Check sheet for the modelled part. Datum: model origin and axes. Units: mm. A direction names the side the tool comes from. Coordinates: 2 decimals unless noted, no trailing zeros. Loops run counter-clockwise (first coordinate to the right, second up) from the corner with the lowest first, then second, coordinate; pieces in that order, holes last. Notation, with made-up numbers: (25.25, 9.25) -> (74.25, 9.25) arc R10 cw to (74.25, 13.25) -> close; hole circle Ø5 at (35, 84.25). An arc over 180 degrees is marked (long way). Use CSV: the item, a comma, the result in double quotes.
```python
from build123d import *

# Parameters (mm, degrees)
SKETCH1_R           = 5.715
SKETCH1_R_2         = 3.175
SKETCH1_W           = 2.54
SKETCH1_H           = 30.48
BOSS_EXTRUDE1_DEPTH = 38.1
SKETCH1_3_R         = 3.175
CUT_EXTRUDE1_DEPTH  = 7.874
SKETCH2_R           = 3.175
CUT_EXTRUDE2_DEPTH  = 15.748
FILLET1_R           = 2.54


with BuildPart() as part:
    # Sketch1 → Boss-Extrude1 (new body, symmetric)
    with BuildSketch(Plane.XY):
        with Locations((0, 38.1)):
            Circle(SKETCH1_R)
        with Locations((0, 38.1)):
            Circle(SKETCH1_R_2, mode=Mode.SUBTRACT)
        with BuildLine():
            Line((0, 30.48), (2.54, 30.48))
            ThreePointArc((2.54, 30.48), (2.925884615, 32.409423077), (4.024171598, 34.042011834))
            ThreePointArc((4.024171598, 34.042011834), (2.351034724, 32.890982749), (0.381023909, 32.39771574))
            ThreePointArc((0.381023909, 32.39771574), (0.096177955, 31.457600747), (0, 30.48))
        make_face()
        with Locations((1.27, 15.24)):
            Rectangle(SKETCH1_W, SKETCH1_H)
    extrude(amount=BOSS_EXTRUDE1_DEPTH, both=True)

    # Sketch1_3 → Cut-Extrude1 (cut, symmetric)
    with BuildSketch(Plane.XY):
        with BuildLine():
            Line((0, 30.48), (2.54, 30.48))
            ThreePointArc((2.54, 30.48), (2.925884615, 32.409423077), (4.024171598, 34.042011834))
            ThreePointArc((4.024171598, 34.042011834), (-2.351034724, 43.309017251), (0.381023909, 32.39771574))
            ThreePointArc((0.381023909, 32.39771574), (0.096177955, 31.457600747), (0, 30.48))
        make_face()
        with Locations((0, 38.1)):
            Circle(SKETCH1_3_R, mode=Mode.SUBTRACT)
    extrude(amount=CUT_EXTRUDE1_DEPTH, both=True, mode=Mode.SUBTRACT)

    # Sketch2 → Cut-Extrude2 (cut)
    with BuildSketch(Plane.XY.offset(38.1)):
        with BuildLine():
            Line((2.54, 30.48), (0, 30.48))
            ThreePointArc((0, 30.48), (0.096177955, 31.457600747), (0.381023909, 32.39771574))
            ThreePointArc((0.381023909, 32.39771574), (-2.351034724, 43.309017251), (4.024171598, 34.042011834))
            ThreePointArc((4.024171598, 34.042011834), (2.925884615, 32.409423077), (2.54, 30.48))
        make_face()
        with Locations((0, 38.1)):
            Circle(SKETCH2_R, mode=Mode.SUBTRACT)
    cut_extrude2 = extrude(amount=-CUT_EXTRUDE2_DEPTH, mode=Mode.SUBTRACT)

    # Mirror1: Cut-Extrude2 across plane
    add(cut_extrude2.mirror(Plane.XY), mode=Mode.SUBTRACT)

    # Fillet1
    fillet1_edges = [part.edges().sort_by_distance(p)[0] for p in [
        (1.27, 0, 38.1),
        (1.27, 30.48, 38.1),
        (1.27, 30.48, -38.1),
        (1.27, 0, -38.1),
    ]]
    fillet(fillet1_edges, radius=FILLET1_R)


solid = part.part
```
1) Draft check along Y on faces 1 (the cylindrical face through (1.252, 29.716, -37.376)), 2 (the cylindrical face through (1.288, 0.724, -37.336)), 3 (the cylindrical face through (-0.69, 35, 15.01)). Enter one of: released by +Y, released by -Y, zero draft, split by the parting line, or undercut.
Answer below:
face 1,"released by +Y"
face 2,"released by -Y"
face 3,"undercut"
2) Cross-section at D-D on z = -7. Record the boundary of the cut face in (x, y), and give its area (3 significant figures).
Answer below:
outline,"(0, 0) -> (2.54, 0) -> (2.54, 30.48) -> (0, 30.48) -> close"
area,"77.4 mm²"
3) Go/stop test with flat-tipped pins: pin 1 Ø1.5 at (y, z) = (33.5, -21.5) entering from +X; pin 2 Ø9 at (y, z) = (21.5, 1) entering from +X; pin 3 Ø6 at (x, z) = (4, 7.5) entering from -Y; pin 4 Ø2 at (x, z) = (1.5, 29) entering from +Y. Record where each tip stops, or that it passes through.
Answer below:
pin 1,"stops at x = 4.22"
pin 2,"stops at x = 2.54"
pin 3,"stops at y = 0"
pin 4,"stops at y = 30.48"
4) Thickness scan on line 1 along X through (y, z) = (38, 19); line 2 along Z through (x, y) = (0.25, 31.5); line 3 along X through (y, z) = (13.5, -19.5). Record the ranges inside material, lowest first. Write a range as from..to.
Answer below:
line 1,"x = -5.71..-3.17, 3.17..5.71"
line 2,"z = -22.35..-7.87, 7.87..22.35"
line 3,"x = 0..2.54"
5) Cross-section at C-C on x = -4. Record the boundary of the cut face in (y, z), and give its area (3 significant figures).
Answer below:
outline,"(34.02, -22.35) -> (42.18, -22.35) -> (42.18, -7.87) -> (34.02, -7.87) -> close; (34.02, 7.87) -> (42.18, 7.87) -> (42.18, 22.35) -> (34.02, 22.35) -> close"
area,"236 mm²"
6) Cross-section at A-A on y = 38.1. Record the boundary of the cut face in (x, z) (3 decimals), and give its area (3 significant figures).
Answer below:
outline,"(-5.715, -22.352) -> (-3.175, -22.352) -> (-3.175, -7.874) -> (-5.715, -7.874) -> close; (-5.715, 7.874) -> (-3.175, 7.874) -> (-3.175, 22.352) -> (-5.715, 22.352) -> close; (3.175, -22.352) -> (5.715, -22.352) -> (5.715, -7.874) -> (3.175, -7.874) -> close; (3.175, 7.874) -> (5.715, 7.874) -> (5.715, 22.352) -> (3.175, 22.352) -> close"
area,"147 mm²"
7) Access from +Z, -Z, +X, -X, +Y, -Y to the whole of each face (thin tool, end or side, straight path). Record for faces 4 (the flat face through (1, 30.48, -29)), 5 (the flat face through (0, 15, 1)), 6 (the flat face through (1, 30.48, 0)).
Answer below:
face 4,"-Z, +X, -X, +Y"
face 5,"+Z, -Z, -X, -Y"
face 6,"+X, -X, +Y"
